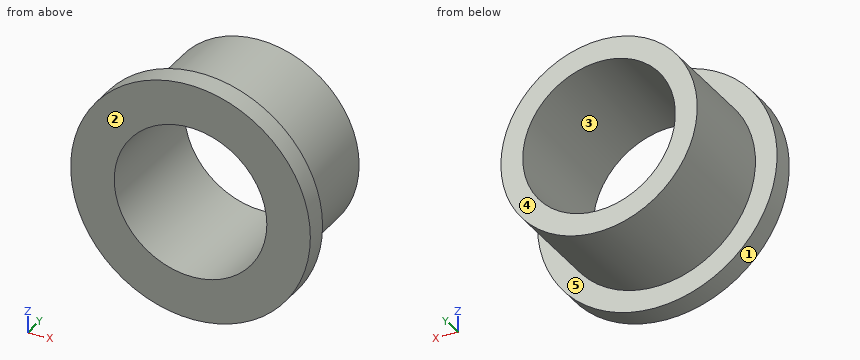
from build123d import *

# Parameters (mm, degrees)
SKETCH2_R           = 9.015
SKETCH2_R_2         = 7.005
BOSS_EXTRUDE1_DEPTH = 14
SKETCH3_R           = 11
SKETCH3_R_2         = 9.015
BOSS_EXTRUDE2_DEPTH = 2
SKETCH4_R           = 9.015
CUT_EXTRUDE1_DEPTH  = 2.475


with BuildPart() as part:
    # Sketch2 → Boss-Extrude1 (new body)
    with BuildSketch(Plane(origin=(0, 0, 0), x_dir=(1, 0, 0), z_dir=(0, 1, 0))):
        Circle(SKETCH2_R)
        Circle(SKETCH2_R_2, mode=Mode.SUBTRACT)
    extrude(amount=BOSS_EXTRUDE1_DEPTH)

    # Sketch3 → Boss-Extrude2 (add)
    with BuildSketch(Plane(origin=(0, 0, 0), x_dir=(1, 0, 0), z_dir=(0, 1, 0))):
        Circle(SKETCH3_R)
        Circle(SKETCH3_R_2, mode=Mode.SUBTRACT)
    extrude(amount=BOSS_EXTRUDE2_DEPTH)

    # Sketch4 → Cut-Extrude1 (cut)
    with BuildSketch(Plane(origin=(0, 14, 0), x_dir=(1, 0, 0), z_dir=(0, 1, 0))):
        Circle(SKETCH4_R)
    extrude(amount=-CUT_EXTRUDE1_DEPTH, mode=Mode.SUBTRACT)


solid = part.part
Check sheet for the modelled part. Datum: model origin and axes. Units: mm. Face numbers are marked on the shaded views. A direction names the side the tool comes from. Round coordinates to 2 decimals unless told otherwise and drop trailing zeros. Loops run counter-clockwise (first coordinate to the right, second up) from the corner with the lowest first, then second, coordinate; pieces in that order, holes last.
1. Sectioned sample at B-B on z = 0. Record the boundary of the cut face in (x, y) (3 decimals), and give its area (3 significant figures).
2. Set-up check for the marked faces 4 and 5: record each of +Z, -Z, +X, -X, +Y, -Y from which the full face is reachable in a straight line by a thin tool's end or side.
3. Sectioned sample at A-A on x = 0. Record the boundary of the cut face in (y, z) (3 decimals).
4. Mould release check, pull along X, two halves, no side actions. Record for the marked faces 1, 2 and 3: released by +X, released by -X, zero draft, split by the parting line, or undercut.
5. Sectioned sample at D-D on z = -8.25. Record the boundary of the cut face in (x, y) (3 decimals).
6. Gauge pin test, flat ends, axial feed: pin 1 Ø1.5 at (x, y) = (1, 4.5) entering from +Z; pin 2 Ø6 at (x, y) = (7, 9) entering from -Z; pin 3 Ø1.5 at (y, z) = (10, 0.5) entering from -X (3 decimals). Record the tip position at first contact, or that the pin passes through.
7. Scan lines: probe 1 along X at (y, z) = (5.25, 0) (3 decimals); probe 2 along Y at (x, z) = (-3.5, 8.75). Record each from-to range of solid material in increasing order.
8. Sectioned sample at C-C on y = 4.5. Record the boundary of the cut face in (x, z) (3 decimals), and give its area (3 significant figures).
Recorded:
1. outline: (-11, 0) - (-7.005, 0) - (-7.005, 11.525) - (-9.015, 11.525) - (-9.015, 2) - (-11, 2) - close; (7.005, 0) - (11, 0) - (11, 2) - (9.015, 2) - (9.015, 11.525) - (7.005, 11.525) - close
1. area: 54.3 mm2
2. face 4: +Z, -Z, +X, -X, +Y
2. face 5: +Y
3. outline: (0, -11) - (2, -11) - (2, -9.015) - (11.525, -9.015) - (11.525, -7.005) - (0, -7.005) - close; (0, 7.005) - (11.525, 7.005) - (11.525, 9.015) - (2, 9.015) - (2, 11) - (0, 11) - close
4. face 1: split by the parting line
4. face 2: zero draft
4. face 3: undercut
5. outline: (-7.276, 0) - (7.276, 0) - (7.276, 2) - (3.634, 2) - (3.634, 11.525) - (-3.634, 11.525) - (-3.634, 2) - (-7.276, 2) - close
6. pin 1: stops at z = 9.01
6. pin 2: stops at z = -8.08
6. pin 3: stops at x = -9.015
7. probe 1: x = -9.015 to -7.005, 7.005 to 9.015
7. probe 2: y = 0 to 2
8. outline: circle Ø18.03 at (0, 0); hole circle Ø14.01 at (0, 0)
8. area: 101 mm2
